Part model, mm, in its own coordinate system. Face numbers are marked on the shaded views. Coordinates: 2 decimals unless noted, no trailing zeros. Loops run counter-clockwise (first coordinate to the right, second up) from the corner with the lowest first, then second, coordinate; pieces in that order, holes last. Notation, with made-up numbers: (74.5, -25) - (91.5, -25) arc R25 ccw to (91.5, 0) - close; hole circle Ø8 at (21.25, -10.75). An arc over 180 degrees is marked (long way). Use a Markdown table: item, result. Add a question column.
1) Band-saw the part on D-D (y = -6.75). Give the cut face in (x, z), plus the area to 3 significant figures.
2) Band-saw the part on C-C (z = 4). Give the cut face in (x, y).
3) Drop flat-ended pins along their axis: P1, Ø2, axis at x = 1.5, y = 6, coming from the -Z side; P2, Ø4, axis at x = 0, y = 1, coming from the -Z side; P3, Ø1.5, axis at y = 5, z = 5.5, coming from the +X side; P4, Ø1.5, axis at y = -4, z = 5, coming from the -X side. Give the stop position or say it passes through.
4) Pull direction Z, two halves, no side cores. Call the marked faces 1, 2, 3 and 4: +Z half, -Z half, draft (parallel to the pull), parting line (faces both ways), or undercut.
5) Band-saw the part on A-A (x = 0). Give the cut face in (y, z), plus the area to 3 significant figures.
6) Probe probe 1 along Y at (x, z) = (0, 2.25); probe 2 along Z at (x, y) = (6.5, -5); probe 3 along Y at (x, z) = (-1, 4). List the from-to ranges inside material, lowest first. Write a range as [from, to].
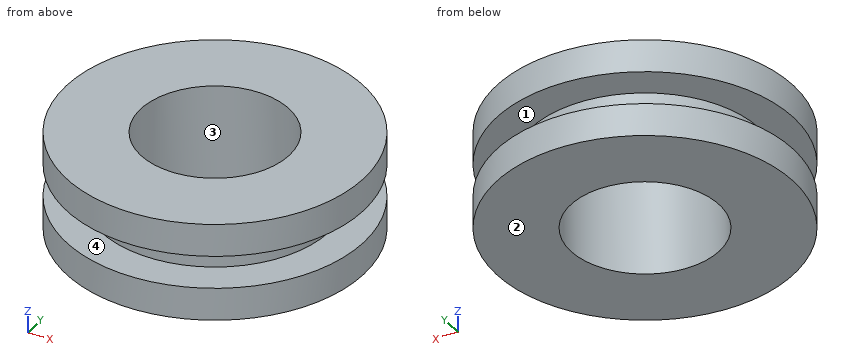
Autodesk Inventor part; units mm, degrees
ref_plane "YZ Plane" through (0, 0, 0) normal (1, 0, 0) x (0, 1, 0)
ref_plane "XZ Plane" through (0, 0, 0) normal (0, 1, 0) x (-1, 0, 0)
ref_plane "XY Plane" through (0, 0, 0) normal (0, 0, 1) x (1, 0, 0)
sketch "Sketch1" plane through (0, 0, 0) normal (0, 0, 1) x (1, 0, 0)
  circle A0 centre (0, 0) radius 5
  circle A1 centre (0, 0) radius 10
  dimension "d0" = 10
  dimension "d1" = 20
extrude "Extrusion1" add sketch "Sketch1" along normal blind 2.2
sketch "Sketch2" plane through (0, 0, 2.2) normal (0, 0, 1) x (1, 0, 0)
  circle A0 centre (0, 0) radius 5
  circle A1 centre (0, 0) radius 10
  circle A2 centre (0, 0) radius 7.7
  dimension "d4" = 15.4
extrude "Extrusion2" add sketch "Sketch2" along normal blind 4.4 contours A2
sketch "Sketch3" plane through (0, 0, 6.6) normal (0, 0, 1) x (1, 0, 0)
  circle A0 centre (0, 0) radius 7.7
  circle A1 centre (0, 0) radius 10
extrude "Extrusion3" add sketch "Sketch3" against normal blind 2.2
properties part number "pulley_wheel" material "Steel"
Answer block:
| question | item | result |
|---|---|---|
| 1 | outline | (-7.38, 0) - (7.38, 0) - (7.38, 2.2) - (3.71, 2.2) - (3.71, 4.4) - (7.38, 4.4) - (7.38, 6.6) - (-7.38, 6.6) - (-7.38, 4.4) - (-3.71, 4.4) - (-3.71, 2.2) - (-7.38, 2.2) - close |
| 1 | area | 81.2 mm2 |
| 2 | outline | circle Ø15.4 at (0, 0); hole circle Ø10 at (0, 0) |
| 3 | P1 | z = 0 |
| 3 | P2 | through |
| 3 | P3 | x = 9.05 |
| 3 | P4 | x = -9.46 |
| 4 | face 1 | undercut |
| 4 | face 2 | -Z half |
| 4 | face 3 | draft |
| 4 | face 4 | undercut |
| 5 | outline | (-10, 0) - (-5, 0) - (-5, 6.6) - (-10, 6.6) - (-10, 4.4) - (-7.7, 4.4) - (-7.7, 2.2) - (-10, 2.2) - close; (5, 0) - (10, 0) - (10, 2.2) - (7.7, 2.2) - (7.7, 4.4) - (10, 4.4) - (10, 6.6) - (5, 6.6) - close |
| 5 | area | 55.9 mm2 |
| 6 | probe 1 | [-7.7, -5], [5, 7.7] |
| 6 | probe 2 | [0, 2.2], [4.4, 6.6] |
| 6 | probe 3 | [-7.63, -4.9], [4.9, 7.63] |
